Autodesk Inventor part; units mm, degrees
ref_plane "YZ Plane" through (0, 0, 0) normal (1, 0, 0) x (0, 1, 0)
ref_plane "XZ Plane" through (0, 0, 0) normal (0, 1, 0) x (-1, 0, 0)
ref_plane "XY Plane" through (0, 0, 0) normal (0, 0, 1) x (1, 0, 0)
sketch "Náčrt1" plane through (0, 0, 0) normal (1, 0, 0) x (0, 1, 0)
  line L0 (14.5, 15) -> (-14.5, 15)
  line L1 (-14.5, 15) -> (-14.5, -15)
  line L2 (-14.5, -15) -> (14.5, -15)
  line L3 (14.5, -15) -> (14.5, 15)
  line L4 (14.5, 5.5) -> (16.6, 5.5)
  line L5 (16.6, 5.5) -> (16.6, -5.5)
  line L6 (16.6, -5.5) -> (14.5, -5.5)
  line L7 (14.5, -5.5) -> (14.5, 5.5)
  point P0 (0, 0)
  dimension "d0" = 29
  dimension "d1" = 30
  dimension "d2" = 2.1
  dimension "d3" = 11
  dimension "d4" = 15
  dimension "d5" = 14.5
  dimension "d6" = 5.5
extrude "Vysunutí1" add sketch "Náčrt1" along normal blind 4
sketch "Náčrt2" plane through (4, 0, 0) normal (1, 0, 0) x (0, 0, -1)
  line L0 (-15, -4.5) -> (15, -4.5)
  line L1 (15, -4.5) -> (15, -11.5)
  line L2 (15, -11.5) -> (-15, -11.5)
  line L3 (-15, -11.5) -> (-15, -4.5)
  line L4 (5.5, 14.5) -> (5.5, 16.6)
  line L5 (5.5, 16.6) -> (-5.5, 16.6)
  line L6 (-5.5, 16.6) -> (-5.5, 14.5)
  line L7 (-5.5, 14.5) -> (-15, 14.5)
  line L8 (-15, 14.5) -> (-15, -14.5)
  line L9 (-15, -14.5) -> (15, -14.5)
  line L10 (15, -14.5) -> (15, 14.5)
  line L11 (15, 14.5) -> (5.5, 14.5)
  line L12 (-15, 14.5) -> (-15, -14.5)
  line L13 (15, -14.5) -> (15, 14.5)
  point P0 (0, 0)
  dimension "d9" = 10
  dimension "d10" = 3
extrude "Vysunutí2" add sketch "Náčrt2" along normal blind 1.2 contours L0 L1 L2 L3
properties part number "gamma"
Check sheet for the modelled part. Datum: model origin and axes. Units: mm. A direction names the side the tool comes from. Give positions to 0.01 mm unless a question says otherwise; leave off trailing zeros. Write each loop counter-clockwise with the first axis right and the second up, starting at its lowest first coordinate (ties: lowest second). Pieces come first, ordered by that corner, then holes.
Item 1: Gauge pin test, flat ends, axial feed: pin 1 (17 mm diameter, centred on y = 9, z = -4, fed in from +X); pin 2 (1.1 mm diameter, centred on x = 1.5, y = 15.5, fed in from +Z); pin 3 (1.1 mm diameter, centred on x = 2.5, y = 15.5, fed in from -Z); pin 4 (1.3 mm diameter, centred on x = 4.5, z = -1.5, fed in from +Y). Record the tip position at first contact, or that the pin passes through.
Item 2: Cross-section at B-B (z = 11.25). Enter the section's corners in (x, y), and give its area (3 significant figures).
Item 3: Cross-section at D-D (x = 4.4). Enter the section's corners in (y, z).
Item 4: Cross-section at C-C (y = 11.5). Enter the section's corners in (x, z).
Item 5: Scan lines: L1, parallel to Y at x = 3.2, z = 7.75; L2, parallel to X at y = -1, z = 6.5; L3, parallel to Y at x = 4.7, z = 9.5. Record each from-to range of solid material in increasing order.
Item 6: Draft check along Z on faces 1 (the face through (2, 16, -5.5)), 2 (the face through (2, 16, 5.5)), 3 (the face through (2, 14.5, -10)). Enter one of: released by +Z, released by -Z, zero draft, split by the parting line, or undercut.
Item 7: Cross-section at A-A (x = 1.05). Enter the section's corners in (y, z).
Item 8: Access from +Z, -Z, +X, -X, +Y, -Y to the whole of each face (thin tool, end or side, straight path). Record for faces 4 (the face through (5.2, -8, 0)), 5 (the face through (2, 14.5, 10)), 6 (the face through (5, -4.5, 0)), 7 (the face through (5, -11.5, 0)).
Report:
1. pin 1: stops at x = 4
1. pin 2: stops at z = 5.5
1. pin 3: stops at z = -5.5
1. pin 4: stops at y = 16.6
2. outline: (0, -14.5) - (4, -14.5) - (4, -11.5) - (5.2, -11.5) - (5.2, -4.5) - (4, -4.5) - (4, 14.5) - (0, 14.5) - close
2. area: 124 mm2
3. outline: (-11.5, -15) - (-4.5, -15) - (-4.5, 15) - (-11.5, 15) - close
4. outline: (0, -15) - (4, -15) - (4, 15) - (0, 15) - close
5. L1: y = -14.5 to 14.5
5. L2: x = 0 to 4
5. L3: y = -11.5 to -4.5
6. face 1: released by -Z
6. face 2: released by +Z
6. face 3: zero draft
7. outline: (-14.5, -15) - (14.5, -15) - (14.5, -5.5) - (16.6, -5.5) - (16.6, 5.5) - (14.5, 5.5) - (14.5, 15) - (-14.5, 15) - close
8. face 4: +Z, -Z, +X, +Y, -Y
8. face 5: +Z, +X, -X, +Y
8. face 6: +Z, -Z, +X, +Y
8. face 7: +Z, -Z, +X, -Y
